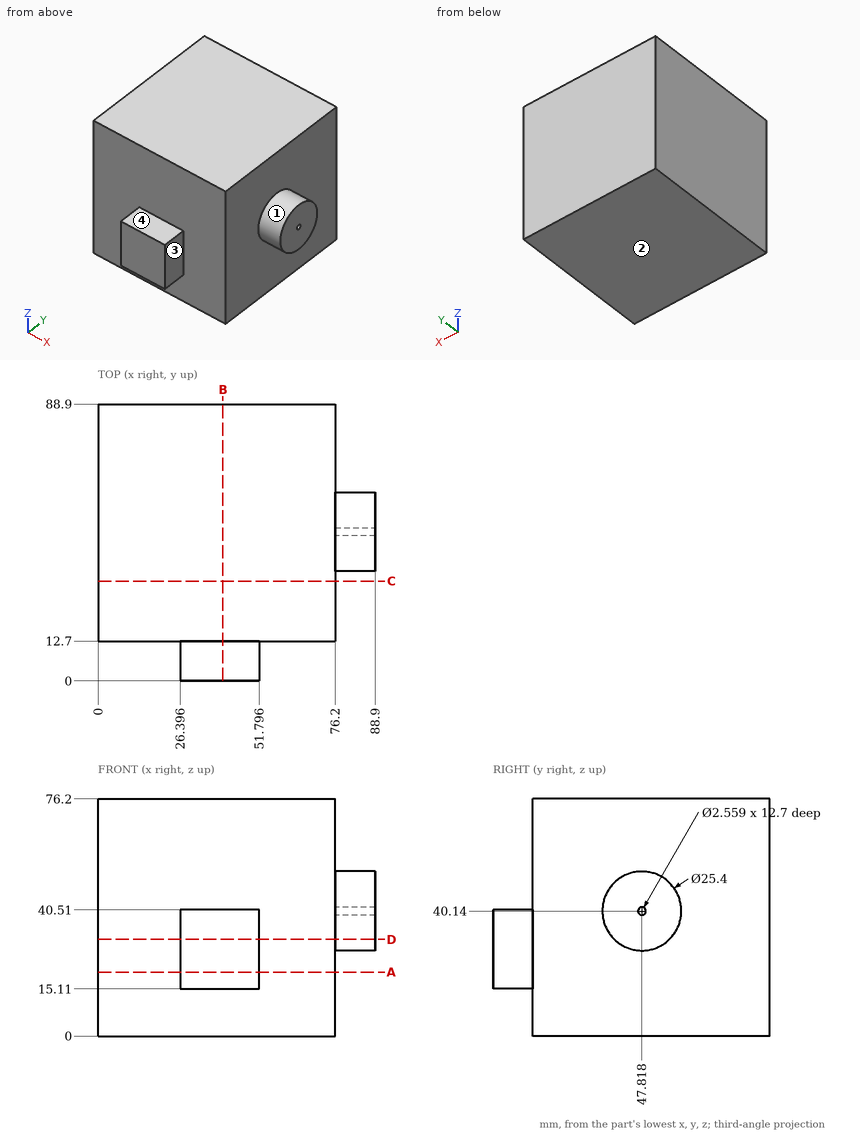
Part print with two shaded views. Sizes in mm from the minimum x, y, z corner. A direction names the side the tool comes from. Round coordinates to 2 decimals unless told otherwise and drop trailing zeros. Write each loop counter-clockwise with the first axis right and the second up, starting at its lowest first coordinate (ties: lowest second). Pieces come first, ordered by that corner, then holes. Notation, with made-up numbers: (16, 6.5) -> (69, 6.5) arc R12 cw to (69, 12.5) -> close; hole circle Ø4 at (-6, -30). An arc over 180 degrees is marked (long way). Use one line per item in the form item = value.
Q1. Drill centre lines: L1, parallel to X at y = 43, z = 27; L2, parallel to Y at x = 60, z = 67; L3, parallel to Y at x = 81, z = 43 (1 decimal). Where is each one in solid material? Low to high.
Conclusion:
L1 = 0 to 76.2
L2 = 12.7 to 88.9
L3 = 35.4 to 60.2
Q2. Band-saw the part on C-C, the plane y = 32. Write the cut outline in (x, z).
Conclusion:
outline = (0, 0) -> (76.2, 0) -> (76.2, 76.2) -> (0, 76.2) -> close
Q3. Band-saw the part on A-A, the plane z = 20.5. Write the cut outline in (x, y) (1 decimal), then the cut area to 3 significant figures.
Conclusion:
outline = (0, 12.7) -> (26.4, 12.7) -> (26.4, 0) -> (51.8, 0) -> (51.8, 12.7) -> (76.2, 12.7) -> (76.2, 88.9) -> (0, 88.9) -> close
area = 6,130 mm²
Q4. Drop flat-ended pins along their axis: P1, Ø6.5, axis at y = 5, z = 22.5, coming from the -X side; P2, Ø0.8, axis at y = 48, z = 39.5, coming from the +X side; P3, Ø6.5, axis at x = 42, y = 9, coming from the -Z side. Give the stop position or say it passes through.
Conclusion:
P1 = 26.4
P2 = 76.2
P3 = 15.11
Q5. Band-saw the part on B-B, the plane x = 40. Write the cut outline in (y, z), then the cut area to 3 significant figures.
Conclusion:
outline = (0, 15.11) -> (12.7, 15.11) -> (12.7, 0) -> (88.9, 0) -> (88.9, 76.2) -> (12.7, 76.2) -> (12.7, 40.51) -> (0, 40.51) -> close
area = 6,130 mm²
Q6. Band-saw the part on D-D, the plane z = 31. Write the cut outline in (x, y) (1 decimal).
Conclusion:
outline = (0, 12.7) -> (26.4, 12.7) -> (26.4, 0) -> (51.8, 0) -> (51.8, 12.7) -> (76.2, 12.7) -> (76.2, 39) -> (88.9, 39) -> (88.9, 56.6) -> (76.2, 56.6) -> (76.2, 88.9) -> (0, 88.9) -> close
Q7. Tool access for the marked faces 1, 2, 3 and 4: list every direction of +Z, -Z, +X, -X, +Y, -Y with a clear straight run to the whole face (end or side of a thin tool).
Conclusion:
face_1 = +X
face_2 = -Z, +X, -X, +Y, -Y
face_3 = +Z, -Z, +X, -Y
face_4 = +Z, +X, -X, -Y
